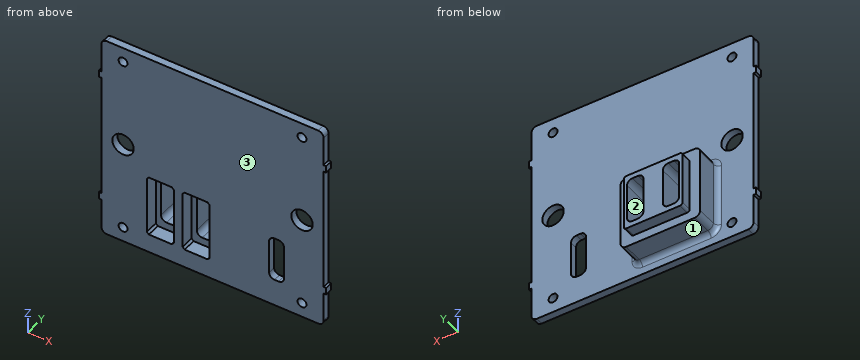
from build123d import *

# Parameters (mm, degrees)
EXTRUDE_1_DEPTH     = 1.5
SKETCH_2_R          = 2.15
SKETCH_2_R_2        = 0.9
CUT_EXTRUDE_1_DEPTH = 32.070444155
SKETCH_3_W          = 12.2
SKETCH_3_H          = 12
EXTRUDE_2_DEPTH     = 7.2
SKETCH_4_W          = 16
SKETCH_4_H          = 15
EXTRUDE_3_DEPTH     = 7.2
SKETCH_5_W          = 3.3
SKETCH_5_H          = 9.3
CUT_EXTRUDE_2_DEPTH = 33.230614329
SKETCH_6_W          = 5.4
SKETCH_6_H          = 12.4
CUT_EXTRUDE_3_DEPTH = 2.7
SKETCH_7_W          = 3
SKETCH_7_H          = 9
CUT_EXTRUDE_4_DEPTH = 33.230614329
SKETCH_8_W          = 16
SKETCH_8_H          = 15
SKETCH_8_W_2        = 11.8
SKETCH_8_H_2        = 11.4
CUT_EXTRUDE_5_DEPTH = 2.2
FILLET_1_R          = 1.1
FILLET_2_R          = 0.5
FILLET_3_R          = 1
CHAMFER_1_SIZE      = 0.4


with BuildPart() as part:
    # 草图1 → 凸台-拉伸1 (new body)
    with BuildSketch(Plane(origin=(0, 0, 0), x_dir=(1, 0, 0), z_dir=(0, 1, 0))):
        Polygon((-22.35, -12.55), (-22.85, -12.55), (-22.85, -13.95), (-22.35, -13.95), (-22.35, -21), (22.35, -21), (22.35, -13.95), (22.85, -13.95), (22.85, -12.55), (22.35, -12.55), (22.35, 12.55), (22.85, 12.55), (22.85, 13.95), (22.35, 13.95), (22.35, 21), (-22.35, 21), (-22.35, 13.95), (-22.85, 13.95), (-22.85, 12.55), (-22.35, 12.55), align=None)
    extrude(amount=EXTRUDE_1_DEPTH)

    # 草图2 → 切除-拉伸1 (cut, through all)
    with BuildSketch(Plane(origin=(0, 1.5, 0), x_dir=(1, 0, 0), z_dir=(0, 1, 0))):
        with Locations(Location((-18, 0, 0), (0, 0, 270))):
            Circle(SKETCH_2_R)
        with Locations(Location((18, 0, 0), (0, 0, 270))):
            Circle(SKETCH_2_R)
        with Locations(Location((-18, -18, 0), (0, 0, 270))):
            Circle(SKETCH_2_R_2)
        with Locations(Location((-18, 18, 0), (0, 0, 270))):
            Circle(SKETCH_2_R_2)
        with Locations(Location((18, -18, 0), (0, 0, 90))):
            Circle(SKETCH_2_R_2)
        with Locations(Location((18, 18, 0), (0, 0, 90))):
            Circle(SKETCH_2_R_2)
    extrude(amount=-CUT_EXTRUDE_1_DEPTH, mode=Mode.SUBTRACT)

    # 草图3 → 凸台-拉伸2 (add)
    with BuildSketch(Plane(origin=(0, 1.5, 0), x_dir=(1, 0, 0), z_dir=(0, 1, 0))):
        with Locations((-6.9, 11)):
            Rectangle(SKETCH_3_W, SKETCH_3_H)
    extrude(amount=EXTRUDE_2_DEPTH)

    # 草图4 → 凸台-拉伸3 (add)
    with BuildSketch(Plane(origin=(0, 1.5, 0), x_dir=(1, 0, 0), z_dir=(0, 1, 0))):
        with Locations((-6.9, 11)):
            Rectangle(SKETCH_4_W, SKETCH_4_H)
    extrude(amount=EXTRUDE_3_DEPTH)

    # 草图5 → 切除-拉伸2 (cut, through all)
    with BuildSketch(Plane(origin=(0, 8.7, 0), x_dir=(1, 0, 0), z_dir=(0, 1, 0))):
        with Locations((-10.5, 11)):
            Rectangle(SKETCH_5_W, SKETCH_5_H)
        with Locations((-3.3, 11)):
            Rectangle(SKETCH_5_W, SKETCH_5_H)
    extrude(amount=-CUT_EXTRUDE_2_DEPTH, mode=Mode.SUBTRACT)

    # 草图6 → 切除-拉伸3 (cut)
    with BuildSketch(Plane.XZ):
        with Locations((-10.5, -11)):
            Rectangle(SKETCH_6_W, SKETCH_6_H)
        with Locations((-3.3, -11)):
            Rectangle(SKETCH_6_W, SKETCH_6_H)
    extrude(amount=-CUT_EXTRUDE_3_DEPTH, mode=Mode.SUBTRACT)

    # 草图7 → 切除-拉伸4 (cut, through all)
    with BuildSketch(Plane.XZ):
        with Locations((12.88, -11)):
            Rectangle(SKETCH_7_W, SKETCH_7_H)
    extrude(amount=-CUT_EXTRUDE_4_DEPTH, mode=Mode.SUBTRACT)

    # 草图8 → 切除-拉伸5 (cut)
    with BuildSketch(Plane(origin=(0, 8.7, 0), x_dir=(1, 0, 0), z_dir=(0, 1, 0))):
        with Locations((-6.9, 11)):
            Rectangle(SKETCH_8_W, SKETCH_8_H)
        with Locations((-6.9, 11)):
            Rectangle(SKETCH_8_W_2, SKETCH_8_H_2, mode=Mode.SUBTRACT)
    extrude(amount=-CUT_EXTRUDE_5_DEPTH, mode=Mode.SUBTRACT)

    # 圆角1
    fillet_1_edges = [part.edges().sort_by_distance(p)[0] for p in [
        (-12.15, 5.7, -15.65),
        (-8.85, 5.7, -15.65),
        (-12.15, 5.7, -6.35),
        (-8.85, 5.7, -6.35),
        (-4.95, 5.7, -15.65),
        (-1.65, 5.7, -15.65),
        (-4.95, 5.7, -6.35),
        (-1.65, 5.7, -6.35),
        (14.38, 0.75, -6.5),
        (14.38, 0.75, -15.5),
        (11.38, 0.75, -15.5),
        (11.38, 0.75, -6.5),
        (-14.9, 4, -3.5),
        (1.1, 4, -3.5),
        (-14.9, 4, -18.5),
        (1.1, 4, -18.5),
        (22.35, 0.75, 21),
        (-22.35, 0.75, 21),
        (-22.35, 0.75, -21),
        (22.35, 0.75, -21),
    ]]
    fillet(fillet_1_edges, radius=FILLET_1_R)

    # 圆角2
    fillet_2_edges = [part.edges().sort_by_distance(p)[0] for p in [
        (-1, 7.6, -5.3),
        (-12.8, 7.6, -5.3),
        (-12.8, 7.6, -16.7),
        (-1, 7.6, -16.7),
    ]]
    fillet(fillet_2_edges, radius=FILLET_2_R)

    # 圆角3
    fillet_3_edges = [part.edges().sort_by_distance(p)[0] for p in [
        (-6.9, 1.5, -18.5),
        (1.1, 1.5, -11),
        (-6.9, 1.5, -3.5),
        (-14.9, 1.5, -11),
        (-14.577817459, 1.5, -3.822182541),
        (-14.577817459, 1.5, -18.177817459),
        (0.777817459, 1.5, -18.177817459),
        (0.777817459, 1.5, -3.822182541),
    ]]
    fillet(fillet_3_edges, radius=FILLET_3_R)

    # 倒角1
    chamfer_1_edges = [part.edges().sort_by_distance(p)[0] for p in [
        (-7.8, 1.35, -4.8),
        (-7.8, 1.35, -17.2),
        (-13.2, 1.35, -17.2),
        (-13.2, 1.35, -4.8),
        (-0.6, 1.35, -4.8),
        (-0.6, 1.35, -17.2),
        (-6, 1.35, -17.2),
        (-6, 1.35, -4.8),
    ]]
    chamfer(chamfer_1_edges, length=CHAMFER_1_SIZE)


solid = part.part
The listing builds one solid part. Answer for the finished solid, in the listing's coordinates (mm). Face numbers are marked on the shaded views. A direction names the side the tool comes from. Give positions to 0.01 mm unless a question says otherwise; leave off trailing zeros. Loops run counter-clockwise (first coordinate to the right, second up) from the corner with the lowest first, then second, coordinate; pieces in that order, holes last. Notation, with made-up numbers: (-9.75, 27.5) - (-5.75, 27.5) arc R15 cw to (-5.75, 34.5) - close; hole circle Ø1 at (3.5, 85). An arc over 180 degrees is marked (long way). Write each question's results on one line, items separated by ' | '.
1. Find section A-A, the plane z = -12. Count the separate pieces of the cut face and the enclosed holes in it, then the cut area to 3 significant figures.
Resolved:
separate pieces: 4 | enclosed holes: 0 | area: 100 mm^2
2. Find section B-B, the plane x = 18. Write down the section's boundary in (y, z).
Resolved:
outline: (0, -21) - (1.5, -21) - (1.5, -18.9) - (0, -18.9) - close; (0, -17.1) - (1.5, -17.1) - (1.5, -2.15) - (0, -2.15) - close; (0, 2.15) - (1.5, 2.15) - (1.5, 17.1) - (0, 17.1) - close; (0, 18.9) - (1.5, 18.9) - (1.5, 21) - (0, 21) - close
3. Consider probe 1 along X at (y, z) = (0.55, -18); probe 2 along X at (y, z) = (7, -11); probe 3 along X at (y, z) = (0.5, -15). Determine where each line is inside the solid, lowest interval first. Write a range as from..to.
Resolved:
probe 1: x = -22.35..-18.9, -17.1..17.1, 18.9..22.35 | probe 2: x = -12.8..-12.15, -8.85..-4.95, -1.65..-1 | probe 3: x = -22.35..-13.2, -7.8..-6, -0.6..11.56, 14.2..22.35
4. Flat-ended cylindrical pins translate along their axes: P1, Ø2, axis at y = 4, z = -8, coming from the -X side; P2, Ø1.4, axis at x = -18, z = 18, coming from the -Y side; P3, Ø0.8, axis at y = 1, z = -11, coming from the +X side; P4, Ø3, axis at x = 1.5, z = 5, coming from the +Y side. Find the tip coordinate at first contact, or state that the pin passes through.
Resolved:
P1: stops at x = -14.9 | P2: passes through | P3: stops at x = 22.35 | P4: stops at y = 1.5
5. Find section D-D, the plane y = 8. Write down the section's boundary in (x, z), then the cut area to 3 significant figures.
Resolved:
outline: (-12.8, -16.2) arc R0.5 ccw to (-12.3, -16.7) - (-1.5, -16.7) arc R0.5 ccw to (-1, -16.2) - (-1, -5.8) arc R0.5 ccw to (-1.5, -5.3) - (-12.3, -5.3) arc R0.5 ccw to (-12.8, -5.8) - close; hole (-12.15, -14.55) arc R1.1 ccw to (-11.05, -15.65) - (-9.95, -15.65) arc R1.1 ccw to (-8.85, -14.55) - (-8.85, -7.45) arc R1.1 ccw to (-9.95, -6.35) - (-11.05, -6.35) arc R1.1 ccw to (-12.15, -7.45) - close; hole (-4.95, -14.55) arc R1.1 ccw to (-3.85, -15.65) - (-2.75, -15.65) arc R1.1 ccw to (-1.65, -14.55) - (-1.65, -7.45) arc R1.1 ccw to (-2.75, -6.35) - (-3.85, -6.35) arc R1.1 ccw to (-4.95, -7.45) - close | area: 75.0 mm^2
6. Find section C-C, the plane z = 0. Write down the section's boundary in (x, y).
Resolved:
outline: (-22.35, 0) - (-20.15, 0) - (-20.15, 1.5) - (-22.35, 1.5) - close; (-15.85, 0) - (15.85, 0) - (15.85, 1.5) - (-15.85, 1.5) - close; (20.15, 0) - (22.35, 0) - (22.35, 1.5) - (20.15, 1.5) - close
7. Which of the six approach directions +Z, -Z, +X, -X, +Y, -Y give full straight-line access (tool end or side, diameter ignored) to the marked faces 1, 2 and 3?
Resolved:
face 1: -Z, +X, -X, +Y | face 2: +Y, -Y | face 3: +Z, -Z, +X, -X, -Y
